Drawing for the job (mm, zero at the part's lowest x, y, z). Coordinates: 2 decimals unless noted, no trailing zeros. Write each loop counter-clockwise with the first axis right and the second up, starting at its lowest first coordinate (ties: lowest second). Pieces come first, ordered by that corner, then holes. Notation, with made-up numbers: M 54,74.25 L 98,74.25 A26 ccw 98,97.25 Z; hole C 25.5,80.25 d4. An arc over 180 degrees is marked long. Put each result on its own line as item: value. Start each with the question number.
Q1. Cut at A-A (x = 85). Write the cut outline in (y, z).
Q2. Cut at C-C (x = 125). Write the cut outline in (y, z).
Q3. Drill centre lines: line 1 along Y through (x, z) = (85, 0.9); line 2 along Z through (x, y) = (83, 198.5); line 3 along Z through (x, y) = (88.5, 55). Where is each one in solid material? Low to high.
Q4. Cut at B-B (z = 85). Write the cut outline in (x, y), then the cut area to 3 significant figures.
Q5. Cut at D-D (z = 105). Write the cut outline in (x, y).
Q6. Drop flat-ended pins along their axis: pin 1 (2 mm diameter, centred on x = 139, y = 351, fed in from +Z); pin 2 (8 mm diameter, centred on y = 86.5, z = 56, fed in from +X); pin 3 (5 mm diameter, centred on y = 192, z = 128, fed in from +X); pin 4 (12 mm diameter, centred on y = 32.7, z = 85, fed in from +X). Give the stop position or say it passes through.
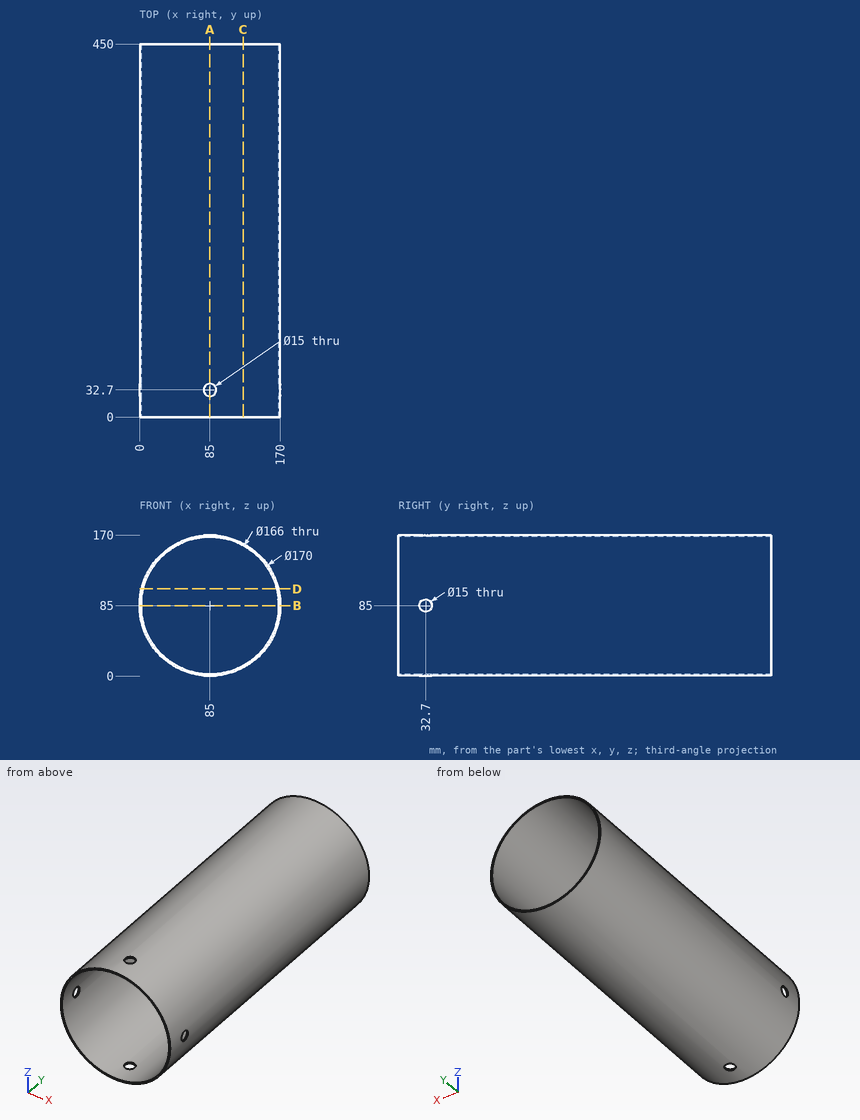
Computed values:
1. outline: M 0,0 L 25.2,0 L 25.2,2 L 0,2 Z; M 0,168 L 25.2,168 L 25.2,170 L 0,170 Z; M 40.2,0 L 450,0 L 450,2 L 40.2,2 Z; M 40.2,168 L 450,168 L 450,170 L 40.2,170 Z
2. outline: M 0,10 L 450,10 L 450,12.27 L 0,12.27 Z; M 0,157.73 L 450,157.73 L 450,160 L 0,160 Z
3. line 1: 0 to 25.2, 40.2 to 450
3. line 2: 0.02 to 2.02, 167.98 to 169.98
3. line 3: 0.07 to 2.07, 167.93 to 169.93
4. outline: M 0,0 L 2,0 L 2,25.2 L 0,25.2 Z; M 0,40.2 L 2,40.2 L 2,450 L 0,450 Z; M 168,0 L 170,0 L 170,25.2 L 168,25.2 Z; M 168,40.2 L 170,40.2 L 170,450 L 168,450 Z
4. area: 1,740 mm2
5. outline: M 2.39,0 L 4.45,0 L 4.45,450 L 2.39,450 Z; M 165.55,0 L 167.61,0 L 167.61,450 L 165.55,450 Z
6. pin 1: z = 151.45
6. pin 2: x = 166.24
6. pin 3: x = 159.73
6. pin 4: through
